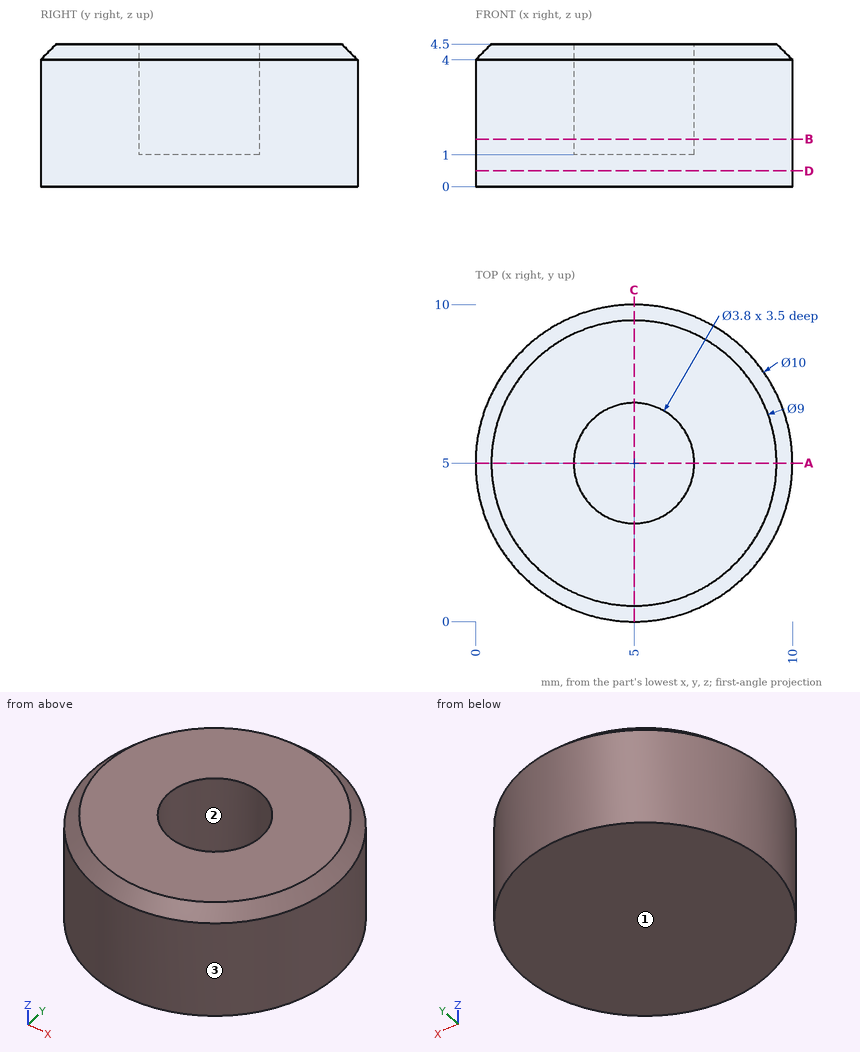
For this review, use the dimensioned drawing (mm, ordinates from the lowest corner) and the shaded views. Round coordinates to 2 decimals unless told otherwise and drop trailing zeros. Order: outer loops, then holes, each group sorted by start corner. A loop starts at its lowest first (then second) coordinate and runs counter-clockwise, first axis right, second up. Notation, with made-up numbers: (6, -6.75) -> (35, -6.75) arc R25 ccw to (35, 20.25) -> close; hole circle Ø6 at (16.25, 62.25). An arc over 180 degrees is marked (long way). One line per item, written item: value. Start each with the question number.
Q1. Take a section at B-B (z = 1.5). Write out the cut boundary in (x, y).
Q2. Take a section at A-A (y = 5). Write out the cut boundary in (x, z).
Q3. Take a section at D-D (z = 0.5). Write out the cut boundary in (x, y).
Q4. Mouldability with a two-part tool opening along X and no side actions: class the marked faces 1, 2 and 3 as released by +X, released by -X, zero draft, split by the parting line, or undercut.
Q5. Clearance check with flat-ended pins moving along their axes: pin 1 Ø2 at (y, z) = (8, 3.5) entering from +X; pin 2 Ø1.5 at (y, z) = (2.5, 3.5) entering from +X. State where each tip first meets the part, or that it passes through.
Q6. Wall thickness on line 1 (Y direction, x = 5, z = 2.45); line 2 (Z direction, x = 4.5, y = 4); line 3 (Y direction, x = 6.5, z = 3.7): over which ranges is each line inside the solid? List them lowest first.
Reported:
1. outline: circle Ø10 at (5, 5); hole circle Ø3.8 at (5, 5)
2. outline: (0, 0) -> (10, 0) -> (10, 4) -> (9.5, 4.5) -> (6.9, 4.5) -> (6.9, 1) -> (3.1, 1) -> (3.1, 4.5) -> (0.5, 4.5) -> (0, 4) -> close
3. outline: circle Ø10 at (5, 5)
4. face 1: zero draft
4. face 2: undercut
4. face 3: split by the parting line
5. pin 1: stops at x = 9.58
5. pin 2: stops at x = 9.68
6. line 1: y = 0 to 3.1, 6.9 to 10
6. line 2: z = 0 to 1
6. line 3: y = 0.23 to 3.83, 6.17 to 9.77
